Design review of the part shown in the three views and the two pictorial views. Dimensions are in mm from the part's minimum x, y and z. A direction names the side the tool comes from. Round coordinates to 2 decimals unless told otherwise and drop trailing zeros. Order: outer loops, then holes, each group sorted by start corner. A loop starts at its lowest first (then second) coordinate and runs counter-clockwise, first axis right, second up.
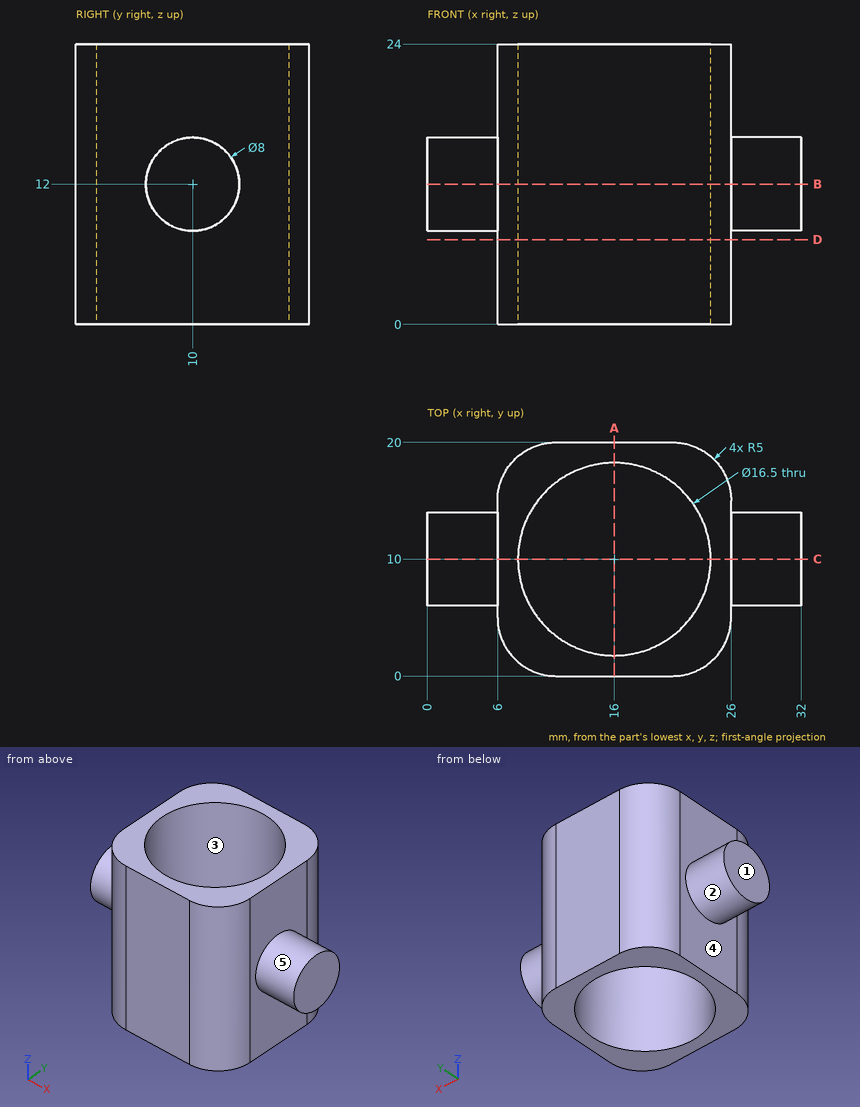
1) The part is to be moulded in two halves that separate along Y. For the marked faces 3, 4 and 5, say which applies: released by +Y, released by -Y, zero draft, split by the parting line, or undercut.
Results:
face 3: undercut
face 4: zero draft
face 5: split by the parting line
2) For the marked faces 1 and 2, list the 3-axis set-ups (+Z, -Z, +X, -X, +Y, -Y) from which the entire face can be reached by the end or side of a thin tool; tool diameter is ignored.
Results:
face 1: +Z, -Z, -X, +Y, -Y
face 2: -X
3) Take a section at B-B on z = 12. Give the boundary of the cut face in (x, y), plus the area to 3 significant figures.
Results:
outline: (0, 6) - (6, 6) - (6, 5) arc R5 ccw to (11, 0) - (21, 0) arc R5 ccw to (26, 5) - (26, 6) - (32, 6) - (32, 14) - (26, 14) - (26, 15) arc R5 ccw to (21, 20) - (11, 20) arc R5 ccw to (6, 15) - (6, 14) - (0, 14) - close; hole circle Ø16.5 at (16, 10)
area: 261 mm2
4) Take a section at D-D on z = 7.25. Give the boundary of the cut face in (x, y).
Results:
outline: (6, 5) arc R5 ccw to (11, 0) - (21, 0) arc R5 ccw to (26, 5) - (26, 15) arc R5 ccw to (21, 20) - (11, 20) arc R5 ccw to (6, 15) - close; hole circle Ø16.5 at (16, 10)
5) Take a section at C-C on y = 10. Give the boundary of the cut face in (x, z).
Results:
outline: (0, 8) - (6, 8) - (6, 0) - (7.75, 0) - (7.75, 24) - (6, 24) - (6, 16) - (0, 16) - close; (24.25, 0) - (26, 0) - (26, 8) - (32, 8) - (32, 16) - (26, 16) - (26, 24) - (24.25, 24) - close
6) To check wall thickness, follow line 1 along Y through (x, z) = (16, 7.5); line 2 along Y through (x, z) = (11, 17.5); line 3 along X through (y, z) = (5.75, 8.5). State the ranges of each line that lie inside material, in increasing order.
Results:
line 1: y = 0 to 1.75, 18.25 to 20
line 2: y = 0 to 3.44, 16.56 to 20
line 3: x = 6 to 8.93, 23.07 to 26
7) Clearance check with a flat-ended pin moving along its axis: P1, Ø6, axis at y = 2, z = 6.5, coming from the -X side. State where the tip first meets the part, or that it passes through.
Results:
P1: stops at x = 6
8) Take a section at A-A on x = 16. Give the boundary of the cut face in (y, z), plus the area to 3 significant figures.
Results:
outline: (0, 0) - (1.75, 0) - (1.75, 24) - (0, 24) - close; (18.25, 0) - (20, 0) - (20, 24) - (18.25, 24) - close
area: 84.0 mm2
